CAD build for the part. Positions are in the model's coordinates, mm. A direction names the side the tool comes from. Coordinates: 2 decimals unless noted, no trailing zeros. Write each loop counter-clockwise with the first axis right and the second up, starting at its lowest first coordinate (ties: lowest second). Pieces come first, ordered by that corner, then holes. Notation, with made-up numbers: (55.25, 31) -> (72.25, 31) arc R35 ccw to (72.25, 64) -> close; hole circle Ø4 at (41, 44). An arc over 180 degrees is marked (long way). Answer as CSV lines item,"result". Start each with the question number.
```python
from build123d import *

# Parameters (mm, degrees)
SKETCH1_W                = 65.08
SKETCH1_H                = 65.08
SKETCH1_W_2              = 60
SKETCH1_H_2              = 60
BOSS_EXTRUDE1_DEPTH      = 25.4
BOSS_EXTRUDE2_DEPTH      = 25.4
BOSS_EXTRUDE2_DEPTH_BACK = 65.08
SKETCH4_W                = 65.08
SKETCH4_H                = 2.54
BOSS_EXTRUDE3_DEPTH      = 25.4
SKETCH5_W                = 60
SKETCH5_H                = 30
BOSS_EXTRUDE4_DEPTH      = 2.54


with BuildPart() as part:
    # Sketch1 → Boss-Extrude1 (new body)
    with BuildSketch(Plane(origin=(0, 0, 0), x_dir=(1, 0, 0), z_dir=(0, 1, 0))):
        with Locations((30, 30)):
            Rectangle(SKETCH1_W, SKETCH1_H)
        with Locations((30, 30)):
            Rectangle(SKETCH1_W_2, SKETCH1_H_2, mode=Mode.SUBTRACT)
    extrude(amount=BOSS_EXTRUDE1_DEPTH)

    # Sketch2 → Boss-Extrude2 (add, two sides: drawn at the far end of the back side and taken through both)
    with BuildSketch(Plane(origin=(0, 0, -62.54), x_dir=(-1, 0, 0), z_dir=(0, 0, -1)).offset(-BOSS_EXTRUDE2_DEPTH_BACK)):
        Polygon((0, 25.4), (0, 55.4), (-60, 55.4), (-60, 25.4), (-62.54, 25.4), (-62.54, 57.94), (2.54, 57.94), (2.54, 25.4), align=None)
    extrude(amount=BOSS_EXTRUDE2_DEPTH + BOSS_EXTRUDE2_DEPTH_BACK)

    # Sketch4 → Boss-Extrude3 (add)
    with BuildSketch(Plane(origin=(0, 0, -62.54), x_dir=(-1, 0, 0), z_dir=(0, 0, -1))):
        with Locations((-30, 24.13)):
            Rectangle(SKETCH4_W, SKETCH4_H)
    extrude(amount=BOSS_EXTRUDE3_DEPTH)

    # Sketch5 → Boss-Extrude4 (add)
    with BuildSketch(Plane.XY.offset(2.54)):
        with Locations((30, 40.4)):
            Rectangle(SKETCH5_W, SKETCH5_H)
    extrude(amount=-BOSS_EXTRUDE4_DEPTH)


solid = part.part
```
1. Cut at D-D (z = -36). Give the cut face in (x, y), then the cut area to 3 significant figures.
2. Cut at A-A (x = 8). Give the cut face in (y, z), then the cut area to 3 significant figures.
3. Tool access for faces 1 (the face through (30, 27, 0)), 2 (the face through (30, 55.4, -43)), 3 (the face through (30, 22.86, -75)), 4 (the face through (60, 28, -34)), 5 (the face through (-2.54, 29, -42)): list every direction of +Z, -Z, +X, -X, +Y, -Y with a clear straight run to the whole face (end or side of a thin tool).
4. Mould opens along X. For faces 6 (the face through (30, 13, -60)), 7 (the face through (62.54, 29, -42)), 8 (the face through (30, 29, 2.54)) say: pulls with the +X half, pulls with the -X half, needs draft (parallel to the pull), parting line crosses it, or undercut.
5. Wall check: line 1 (Z direction, x = 17, y = 6); line 2 (Y direction, x = 22, z = -64); line 3 (X direction, y = 45.5, z = -68). Give the ranges that are in metal, low to high.
6. Cut at B-B (y = 47.5). Give the cut face in (x, z), then the cut area to 3 significant figures.
7. Flat gauge pins, fed straight in: P1, Ø3, axis at x = 42, y = 35.5, coming from the -Z side; P2, Ø1.5, axis at x = 8.5, z = -44.5, coming from the -Y side; P3, Ø25, axis at x = 43.5, y = 12, coming from the -Z side. Where does each tip first touch, or does it go through?
8. Cut at C-C (z = -81.5). Give the cut face in (x, y), then the cut area to 3 significant figures.
Geometry check:
1,outline,"(-2.54, 0) -> (0, 0) -> (0, 55.4) -> (60, 55.4) -> (60, 0) -> (62.54, 0) -> (62.54, 57.94) -> (-2.54, 57.94) -> close"
1,area,"447 mm²"
2,outline,"(0, -62.54) -> (22.86, -62.54) -> (22.86, -87.94) -> (25.4, -87.94) -> (25.4, -60) -> (0, -60) -> close; (0, 0) -> (55.4, 0) -> (55.4, -87.94) -> (57.94, -87.94) -> (57.94, 2.54) -> (0, 2.54) -> close"
2,area,"500 mm²"
3,face 1,"-Y"
3,face 2,"-Z"
3,face 3,"-Z, +X, -X, -Y"
3,face 4,"none"
3,face 5,"+Z, -Z, -X, +Y, -Y"
4,face 6,"undercut"
4,face 7,"pulls with the +X half"
4,face 8,"needs draft"
5,line 1,"-62.54 to -60, 0 to 2.54"
5,line 2,"22.86 to 25.4, 55.4 to 57.94"
5,line 3,"-2.54 to 0, 60 to 62.54"
6,outline,"(-2.54, -87.94) -> (0, -87.94) -> (0, 0) -> (60, 0) -> (60, -87.94) -> (62.54, -87.94) -> (62.54, 2.54) -> (-2.54, 2.54) -> close"
6,area,"612 mm²"
7,P1,"z = 0"
7,P2,"y = 55.4"
7,P3,"z = -87.94"
8,outline,"(-2.54, 22.86) -> (62.54, 22.86) -> (62.54, 57.94) -> (-2.54, 57.94) -> close; hole (0, 25.4) -> (60, 25.4) -> (60, 55.4) -> (0, 55.4) -> close"
8,area,"483 mm²"
